For this review, take the finished solid that the model builds, in its own axes (mm). A direction names the side the tool comes from. Round coordinates to 2 decimals unless told otherwise and drop trailing zeros. Order: outer loops, then holes, each group sorted by start corner. A loop starts at its lowest first (then second) coordinate and runs counter-clockwise, first axis right, second up. Notation, with made-up numbers: (13, -15.75) - (52, -15.75) arc R20 cw to (52, 17.25) - close; hole circle Ø9 at (87.25, 61.25). An arc over 180 degrees is marked (long way). One line per question, with ' | ' between items.
```python
from build123d import *

# Parameters (mm, degrees)
SKETCH1_W           = 218
SKETCH1_H           = 218
SKETCH1_R           = 101.6
BOSS_EXTRUDE1_DEPTH = 38.1
SKETCH2_W           = 25.4
SKETCH2_H           = 25.4
BOSS_EXTRUDE2_DEPTH = 50.8
SKETCH3_W           = 218
SKETCH3_H           = 218
SKETCH3_R           = 101.6
BOSS_EXTRUDE3_DEPTH = 108.6
SKETCH4_W           = 218
SKETCH4_H           = 218
SKETCH4_R           = 92.5
BOSS_EXTRUDE4_DEPTH = 8
CUT_EXTRUDE1_REACH  = 258.89
SKETCH5_W           = 16.393750096
SKETCH5_H           = 25.4


with BuildPart() as part:
    # Sketch1 → Boss-Extrude1 (new body)
    with BuildSketch(Plane(origin=(0, 0, 0), x_dir=(1, 0, 0), z_dir=(0, 1, 0))):
        Rectangle(SKETCH1_W, SKETCH1_H)
        with Locations(Location((0, 0, 0), (0, 0, 90))):
            Circle(SKETCH1_R, mode=Mode.SUBTRACT)
    extrude(amount=BOSS_EXTRUDE1_DEPTH)

    # Sketch2 → Boss-Extrude2 (add)
    with BuildSketch(Plane(origin=(0, 38.1, 0), x_dir=(1, 0, 0), z_dir=(0, 1, 0))):
        with Locations((-96.3, 96.3)):
            Rectangle(SKETCH2_W, SKETCH2_H)
        with Locations((96.3, 96.3)):
            Rectangle(SKETCH2_W, SKETCH2_H)
        with Locations((96.3, -96.3)):
            Rectangle(SKETCH2_W, SKETCH2_H)
        with Locations((-96.3, -96.3)):
            Rectangle(SKETCH2_W, SKETCH2_H)
    extrude(amount=BOSS_EXTRUDE2_DEPTH)

    # Sketch3 → Boss-Extrude3 (add)
    with BuildSketch(Plane(origin=(0, 88.9, 0), x_dir=(1, 0, 0), z_dir=(0, 1, 0))):
        Rectangle(SKETCH3_W, SKETCH3_H)
        with Locations(Location((0, 0, 0), (0, 0, 90))):
            Circle(SKETCH3_R, mode=Mode.SUBTRACT)
    extrude(amount=BOSS_EXTRUDE3_DEPTH)

    # Sketch4 → Boss-Extrude4 (add)
    with BuildSketch(Plane(origin=(0, 197.5, 0), x_dir=(1, 0, 0), z_dir=(0, 1, 0))):
        Rectangle(SKETCH4_W, SKETCH4_H)
        with Locations(Location((0, 0, 0), (0, 0, 270))):
            Circle(SKETCH4_R, mode=Mode.SUBTRACT)
    extrude(amount=BOSS_EXTRUDE4_DEPTH)

    # Sketch5 → Cut-Extrude1 (cut, up to next)
    with BuildSketch(Plane.XZ, mode=Mode.PRIVATE) as cut_extrude1_sk1:
        with Locations((109, 0)):
            Rectangle(SKETCH5_W, SKETCH5_H)
    cut_extrude1_tool1 = extrude(cut_extrude1_sk1.sketch, amount=-CUT_EXTRUDE1_REACH, mode=Mode.PRIVATE) & part.part
    add(cut_extrude1_tool1.solids().sort_by_distance((109, 0, 0))[0], mode=Mode.SUBTRACT)


solid = part.part
```
(1) We need section C-C on x = 0. State the section outline as (y, z) points.
Output values:
outline: (0, -109) - (38.1, -109) - (38.1, -101.6) - (0, -101.6) - close; (0, 101.6) - (38.1, 101.6) - (38.1, 109) - (0, 109) - close; (88.9, -109) - (205.5, -109) - (205.5, -92.5) - (197.5, -92.5) - (197.5, -101.6) - (88.9, -101.6) - close; (88.9, 101.6) - (197.5, 101.6) - (197.5, 92.5) - (205.5, 92.5) - (205.5, 109) - (88.9, 109) - close
(2) We need section A-A on z = 0. State the section outline as (x, y) points, plus the area to 3 significant figures.
Output values:
outline: (-109, 0) - (-101.6, 0) - (-101.6, 38.1) - (-109, 38.1) - close; (-109, 88.9) - (-101.6, 88.9) - (-101.6, 197.5) - (-92.5, 197.5) - (-92.5, 205.5) - (-109, 205.5) - close; (92.5, 197.5) - (101.6, 197.5) - (101.6, 88.9) - (109, 88.9) - (109, 205.5) - (92.5, 205.5) - close | area: 2,150 mm^2
(3) We need section B-B on y = 63.5. State the section outline as (x, z) points, plus the area to 3 significant figures.
Output values:
outline: (-109, -109) - (-83.6, -109) - (-83.6, -83.6) - (-109, -83.6) - close; (-109, 83.6) - (-83.6, 83.6) - (-83.6, 109) - (-109, 109) - close; (83.6, -109) - (109, -109) - (109, -83.6) - (83.6, -83.6) - close; (83.6, 83.6) - (109, 83.6) - (109, 109) - (83.6, 109) - close | area: 2,580 mm^2
(4) Mouldability with a two-part tool opening along Z and no side actions: class faces 4 (the cylindrical face through (-101.51, 18.78, -4.29)), 5 (the flat face through (83.6, 63, -96)), 6 (the flat face through (-2, 101, -109)) as released by +Z, released by -Z, zero draft, split by the parting line, or undercut.
Output values:
face 4: undercut | face 5: zero draft | face 6: released by -Z
(5) For probe 1 along Z at (x, y) = (0, 22); probe 2 along X at (y, z) = (203, 0); probe 3 along Y at (x, z) = (-53, -88.5), list the stretches that pass through material, from the lowest coordinate up. Write a range as [from, to].
Output values:
probe 1: [-109, -101.6], [101.6, 109] | probe 2: [-109, -92.5], [92.5, 109] | probe 3: [0, 38.1], [88.9, 205.5]
(6) For faces 1 (the flat face through (-83.6, 63, -96)), 2 (the flat face through (105, 19, -12.7)), 3 (the flat face through (96, 63, 83.6)), list the 3-axis set-ups (+Z, -Z, +X, -X, +Y, -Y) from which the entire face can be reached by the end or side of a thin tool; tool diameter is ignored.
Output values:
face 1: +Z, -Z | face 2: +X, -Y | face 3: +X, -X
(7) We need section D-D on z = 87. State the section outline as (x, y) points.
Output values:
outline: (-109, 0) - (-52.47, 0) - (-52.47, 38.1) - (-83.6, 38.1) - (-83.6, 88.9) - (-52.47, 88.9) - (-52.47, 197.5) - (-31.42, 197.5) - (-31.42, 205.5) - (-109, 205.5) - close; (31.42, 197.5) - (52.47, 197.5) - (52.47, 88.9) - (83.6, 88.9) - (83.6, 38.1) - (52.47, 38.1) - (52.47, 0) - (109, 0) - (109, 205.5) - (31.42, 205.5) - close
